Here's how the part is built. I have some questions about the finished solid (model axes, mm). A direction names the side the tool comes from. Round coordinates to 2 decimals unless told otherwise and drop trailing zeros. Loops run counter-clockwise (first coordinate to the right, second up) from the corner with the lowest first, then second, coordinate; pieces in that order, holes last. Notation, with made-up numbers: (41.5, -20.5) -> (98.5, -20.5) arc R26 cw to (98.5, 8.5) -> close; hole circle Ø6 at (16.5, -29). An arc over 180 degrees is marked (long way). Use one line per item in the form item = value. Start each with the question number.
Item 1: If I drill on L1, parallel to Z at x = -17, y = -3 (3 decimals); L2, parallel to X at y = -9, z = -2; L3, parallel to Z at x = 19.5, y = -13.5, over which ranges is the centre line in solid material (lowest first)? Write a range as [from, to].
Item 2: For faces 1 (the face through (25, -16, -0.794)), 2 (the face through (0, -16, 28.575)), 3 (the face through (1.52, -15.653, -15.802)), which set-ups out of +Z, -Z, +X, -X, +Y, -Y let a thin tool reach every point of the face, with its end or its side?
Item 3: Thinking about a two-plate mould opening in X: for faces 4 (the face through (-19.05, -16, 0)), 5 (the face through (24, -16, 0.794)), 6 (the face through (28.7, -15.65, -16.96)), which applies, released by +X, released by -X, zero draft, split by the parting line, or undercut?
Item 4: I'm going to push flat-ended pins straight in: pin 1 Ø4 at (x, z) = (-19, 2) entering from +Y; pin 2 Ø1 at (y, z) = (-13, 13.5) entering from +X; pin 3 Ø2 at (y, z) = (-15, -13.5) entering from +X; pin 4 Ø10 at (y, z) = (-26.5, -6.5) entering from -X. Where does each tip first touch, or does it pass through?
Item 5: If we section it at B-B (z = -4): Write out the boundary of the cut face in (x, y), then the cut area to 3 significant figures.
Item 6: If we section it at A-A (x = 26.5): Write out the boundary of the cut face in (y, z), then the cut area to 3 significant figures.
Item 7: If we section it at D-D (x = 6): Write out the boundary of the cut face in (y, z) (3 decimals).
```python
from build123d import *

# Parameters (mm, degrees)
F1_DEPTH = 31.75
F3_DEPTH = 28.575


with BuildPart() as f1:
    # F0 (on Front) → F1 (new body)
    with BuildSketch(Plane.XZ):
        with BuildLine():
            Line((15.855144, 0.79375), (33.328049, 0.79375))
            ThreePointArc((33.328049, 0.79375), (28.81838, 16.75977), (17.171438, 28.575))
            Line((17.171438, 28.575), (-17.171438, 28.575))
            ThreePointArc((-17.171438, 28.575), (-33.3375, 0), (-17.171438, -28.575))
            Line((-17.171438, -28.575), (17.171438, -28.575))
            ThreePointArc((17.171438, -28.575), (28.81838, -16.75977), (33.328049, -0.79375))
            Line((33.328049, -0.79375), (15.855144, -0.79375))
            ThreePointArc((15.855144, -0.79375), (1.200092, -15.829574), (-15.55426, -3.175))
            Line((-15.55426, -3.175), (-19.05, -3.175))
            Line((-19.05, -3.175), (-19.05, 3.175))
            Line((-19.05, 3.175), (-15.55426, 3.175))
            ThreePointArc((-15.55426, 3.175), (1.200092, 15.829574), (15.855144, 0.79375))
        make_face()
    extrude(amount=F1_DEPTH)

    # F2 (on Top) → F3 (cut, symmetric)
    with BuildSketch(Plane.XY):
        Polygon((-20.6375, 0), (-20.6375, 6.484366), (-46.338774, 6.484366), (-45.356732, -28.783964), (-40.792249, -28.783964), align=None)
    extrude(amount=F3_DEPTH, both=True, mode=Mode.SUBTRACT)


solid = f1.part
```
Values found:
q1.L1 = [-28.575, -3.175], [3.175, 28.575]
q1.L2 = [-26.94, -19.05], [15.75, 33.28]
q1.L3 = [-27.04, -0.79], [0.79, 27.04]
q2.face_1 = +X, +Y, -Y
q2.face_2 = +Z, +X, -X, +Y, -Y
q2.face_3 = +Y, -Y
q3.face_4 = undercut
q3.face_5 = zero draft
q3.face_6 = released by +X
q4.pin_1 = 0
q4.pin_2 = 30.7
q4.pin_3 = 30.91
q4.pin_4 = -33.3
q5.outline = (-33.1, -31.75) -> (-15.36, -31.75) -> (-15.36, 0) -> (-20.64, 0) -> (-33.1, -17.79) -> close; (15.36, -31.75) -> (33.1, -31.75) -> (33.1, 0) -> (15.36, 0) -> close
q5.area = 1,020 mm2
q6.outline = (-31.75, -20.23) -> (0, -20.23) -> (0, -0.79) -> (-31.75, -0.79) -> close; (-31.75, 0.79) -> (0, 0.79) -> (0, 20.23) -> (-31.75, 20.23) -> close
q6.area = 1,230 mm2
q7.outline = (-31.75, -28.575) -> (0, -28.575) -> (0, -14.697) -> (-31.75, -14.697) -> close; (-31.75, 14.697) -> (0, 14.697) -> (0, 28.575) -> (-31.75, 28.575) -> close
